Part model, mm, in its own coordinate system. A direction names the side the tool comes from. Give positions to 0.01 mm unless a question says otherwise; leave off trailing zeros. Write each loop counter-clockwise with the first axis right and the second up, starting at its lowest first coordinate (ties: lowest second). Pieces come first, ordered by that corner, then holes. Notation, with made-up numbers: (85.5, 7) - (98.5, 7) arc R25 cw to (98.5, 28) - close; hole circle Ø6 at (11.5, 61.25). An arc over 180 degrees is marked (long way). Answer in a Markdown table with one row per item. Add a question column.
1. Which spindle directions (+Z, -Z, +X, -X, +Y, -Y) get a long thin tool onto all of the face, cutting with end or side? Do faces 4 (the flat face through (-35, 0, 26)), 5 (the flat face through (-17, 0, -10)), 6 (the cylindrical face through (-10.14, 0.596, -2.685)), 7 (the flat face through (-17, 11, 0)), 8 (the flat face through (-17, -7.5, -5)). Say none if no direction does.
2. Probe line 1 along Z through (x, y) = (-10, 0); line 2 along Z through (x, y) = (-22, 5); line 3 along Y through (x, z) = (-26, 9.5). List the from-to ranges inside material, lowest first.
3. Band-saw the part on C-C on x = -33. Write the cut outline in (y, z), plus the area to 3 significant figures.
4. Band-saw the part on B-B on z = 5. Write the cut outline in (x, y).
5. Band-saw the part on A-A on x = -2.5. Write the cut outline in (y, z), plus the area to 3 significant figures.
6. Pull direction Y, two halves, no side cores. Call faces 1 (the cylindrical face through (-18, 6, 15)), 2 (the flat face through (-12, -15, 15)), 3 (the flat face through (-17, 0, 30)): released by +Y, released by -Y, zero draft, split by the parting line, or undercut.
7. Band-saw the part on D-D on z = 15. Write the cut outline in (x, y), plus the area to 3 significant figures.
8. Drop a flat-ended pin along its axis: pin 1 Ø1.5 at (x, y) = (-6.5, 10) entering from -Z. Give the stop position or say it passes through.
```python
from build123d import *

# Parameters (mm, degrees)
F1_DEPTH       = 35
F3_D           = 12
F3_CSINK_D     = 14
F3_CSINK_ANGLE = 90
F4_T1_DEPTH    = 80
F5_D           = 5.5
F5_DEPTH       = 20
F5_TIP         = 1.6523667023


# Not quite as in the source:
# - a fillet or chamfer that OpenCascade refuses, or shapes differently, is made with other operations: its cross-section is extruded or revolved along the edge and cut away or added


with BuildPart() as f1:
    # F0 (on Right) → F1 (new body)
    with BuildSketch(Plane.YZ):
        Polygon((15, 30), (0, 30), (-15, 30), (-15, 0), (-7.5, 0), (-7.5, -10), (0, -10), (7.5, -10), (7.5, 0), (15, 0), align=None)
    extrude(amount=-F1_DEPTH)

    # F3 (through all)
    with Locations(Plane.YZ):
        with Locations((0, 15)):
            CounterSinkHole(F3_D / 2, F3_CSINK_D / 2, counter_sink_angle=F3_CSINK_ANGLE)

    # F4: fillet of radius 10 on 2 edges, made by hand

    # F4_s2 → F4_t1 (cut)
    with BuildSketch(Plane.XY.offset(-25)):
        with BuildLine():
            ThreePointArc((-25, 15), (-32.0710678119, 12.0710678119), (-35, 5))
            Line((-35, 5), (-35, 15))
            Line((-35, 15), (-25, 15))
        make_face()
        with BuildLine():
            ThreePointArc((-35, -5), (-32.0710678119, -12.0710678119), (-25, -15))
            Line((-25, -15), (-35, -15))
            Line((-35, -15), (-35, -5))
        make_face()
    extrude(amount=F4_T1_DEPTH, mode=Mode.SUBTRACT)

    # F5
    with Locations(Plane.YZ):
        with Locations((0, 0)):
            Hole(F5_D / 2, depth=F5_DEPTH)
            with Locations((0, 0, -(F5_DEPTH + F5_TIP / 2))):  # 118° drill point
                Cone(0, F5_D / 2, F5_TIP, mode=Mode.SUBTRACT)


solid = f1.part
```
Values:
| question | item | result |
|---|---|---|
| 1 | face 4 | +Z, -Z, -X, +Y, -Y |
| 1 | face 5 | -Z, +X, -X, +Y, -Y |
| 1 | face 6 | +X |
| 1 | face 7 | -Z, +X, -X, +Y |
| 1 | face 8 | -Z, +X, -X, -Y |
| 2 | line 1 | z = -10 to -2.75, 2.75 to 9, 21 to 30 |
| 2 | line 2 | z = -10 to 11.68, 18.32 to 30 |
| 2 | line 3 | y = -14.95 to -2.4, 2.4 to 14.95 |
| 3 | outline | (-11, 0) - (-7.5, 0) - (-7.5, -10) - (7.5, -10) - (7.5, 0) - (11, 0) - (11, 30) - (-11, 30) - close; hole circle Ø12 at (0, 15) |
| 3 | area | 697 mm² |
| 4 | outline | (-35, -5) arc R10 ccw to (-25, -15) - (0, -15) - (0, 15) - (-25, 15) arc R10 ccw to (-35, 5) - close |
| 5 | outline | (-15, 0) - (-7.5, 0) - (-7.5, -10) - (7.5, -10) - (7.5, 0) - (15, 0) - (15, 30) - (-15, 30) - close; hole circle Ø12 at (0, 15); hole circle Ø5.5 at (0, 0) |
| 5 | area | 913 mm² |
| 6 | face 1 | undercut |
| 6 | face 2 | released by -Y |
| 6 | face 3 | zero draft |
| 7 | outline | (-34.95, -6) arc R10 ccw to (-25, -15) - (0, -15) - (0, -7) - (-1, -6) - close; (-34.95, 6) - (-1, 6) - (0, 7) - (0, 15) - (-25, 15) arc R10 ccw to start |
| 7 | area | 586 mm² |
| 8 | pin 1 | stops at z = 0 |
